Study the drawing (mm; zero at the part's minimum x, y, z) and answer. A direction names the side the tool comes from. Round coordinates to 2 decimals unless told otherwise and drop trailing zeros. Order: outer loops, then holes, each group sorted by start corner. A loop starts at its lowest first (then second) coordinate and runs counter-clockwise, first axis right, second up. Notation, with made-up numbers: (60, 50.5) - (66, 50.5) arc R24 ccw to (66, 80.5) - close; hole circle Ø5 at (-29, 58). An arc over 180 degrees is marked (long way). Use one line per item in the form item = value. Start each with the question number.
Q1. The part is cut by section B-B on y = 62.5. Determine the outline of the cut face in (x, z).
Q2. Given P1, Ø2, axis at x = 13, y = 15.5, coming from the +Z side; P2, Ø2, axis at y = 35.5, z = 91, coming from the +X side; P3, Ø12, axis at x = 15, z = 42.5, coming from the +Y side; P4, Ø6, axis at x = 13, z = 104, coming from the -Y side, each flat-ended and moving along its own axis, determine where each tip first touches the part or whether it passes through.
Q3. Which of the six approach directions +Z, -Z, +X, -X, +Y, -Y give full straight-line access (tool end or side, diameter ignored) to the marked faces 1 and 2?
Q4. The part is cut by section A-A on z = 17.5. Determine the outline of the cut face in (x, y), plus the area to 3 significant figures.
Q5. Find the intervals of material crossed by line 1 (X direction, y = 51, z = 27); line 2 (Z direction, x = 20.5, y = 34.5); line 3 (Z direction, x = 2.75, y = 17.5), in increasing order. Write a range as [from, to].
Q6. The part is cut by section D-D on x = 8.5. Determine the outline of the cut face in (y, z).
Q7. The part is cut by section C-C on y = 40. Determine the outline of the cut face in (x, z), plus the area to 3 significant figures.
Q8. For a pull along X with two mould halves and no side action, classify the marked faces 3, 4, 5 and 6 as +X half, -X half, draft (parallel to the pull), parting line (faces both ways), or undercut.
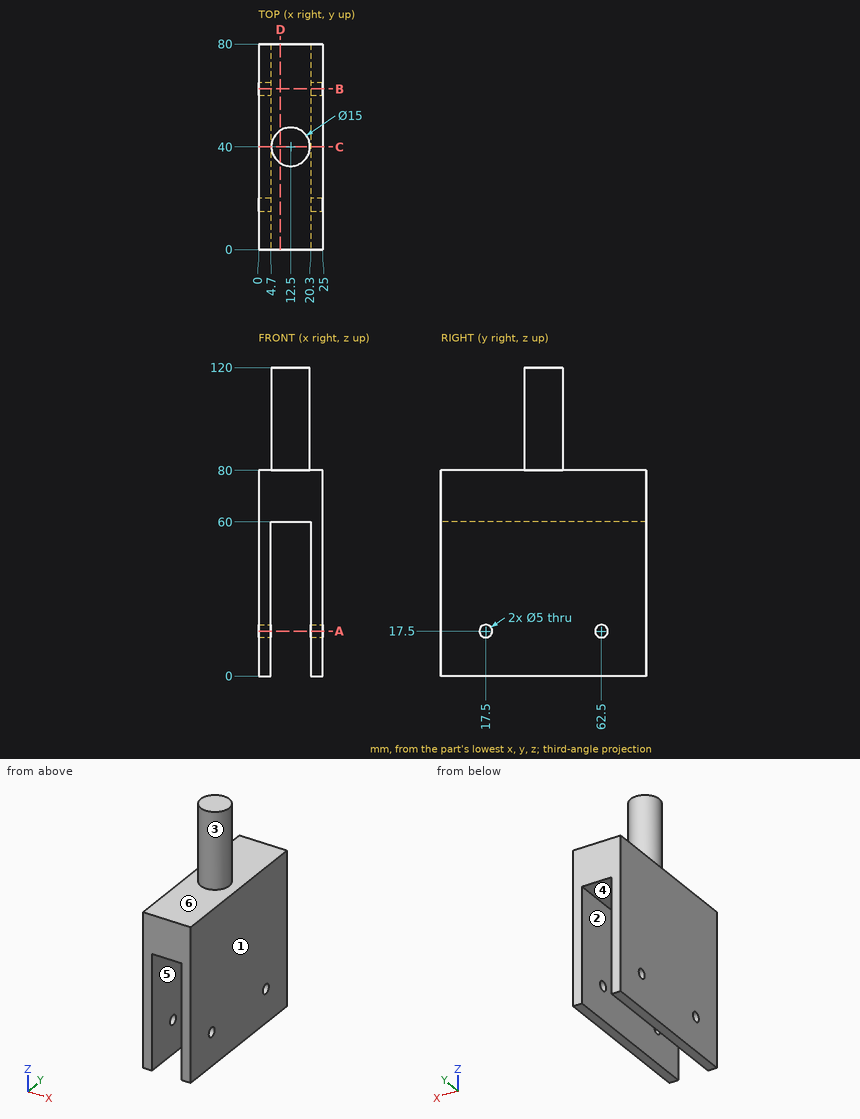
Found:
q1.outline = (0, 0) - (4.7, 0) - (4.7, 15) - (0, 15) - close; (0, 20) - (4.7, 20) - (4.7, 60) - (20.3, 60) - (20.3, 20) - (25, 20) - (25, 80) - (0, 80) - close; (20.3, 0) - (25, 0) - (25, 15) - (20.3, 15) - close
q2.P1 = 80
q2.P2 = 19.13
q2.P3 = 80
q2.P4 = 32.5
q3.face_1 = +Z, -Z, +X, +Y, -Y
q3.face_2 = -Z, +Y, -Y
q4.outline = (0, 0) - (4.7, 0) - (4.7, 15) - (0, 15) - close; (0, 20) - (4.7, 20) - (4.7, 60) - (0, 60) - close; (0, 65) - (4.7, 65) - (4.7, 80) - (0, 80) - close; (20.3, 0) - (25, 0) - (25, 15) - (20.3, 15) - close; (20.3, 20) - (25, 20) - (25, 60) - (20.3, 60) - close; (20.3, 65) - (25, 65) - (25, 80) - (20.3, 80) - close
q4.area = 658 mm²
q5.line_1 = [0, 4.7], [20.3, 25]
q5.line_2 = [0, 80]
q5.line_3 = [0, 15], [20, 80]
q6.outline = (0, 60) - (80, 60) - (80, 80) - (46.34, 80) - (46.34, 120) - (33.66, 120) - (33.66, 80) - (0, 80) - close
q7.outline = (0, 0) - (4.7, 0) - (4.7, 60) - (20.3, 60) - (20.3, 0) - (25, 0) - (25, 80) - (20, 80) - (20, 120) - (5, 120) - (5, 80) - (0, 80) - close
q7.area = 1,660 mm²
q8.face_3 = parting line
q8.face_4 = undercut
q8.face_5 = undercut
q8.face_6 = draft
